Input: part model. Units: mm. Frame: model coordinates. Coordinates: 2 decimals unless noted, no trailing zeros. Loops run counter-clockwise (first coordinate to the right, second up) from the corner with the lowest first, then second, coordinate; pieces in that order, holes last. Notation, with made-up numbers: (71.5, 4) -> (97.5, 4) arc R22 cw to (97.5, 43) -> close; hole circle Ø3 at (-28.5, 8). An arc over 180 degrees is marked (long way). Put each result on its own line as item: value. Start each with the question number.
1) Cut plane B-B (z = 32). Return the cut outline in (x, y), plus the area to 3 significant figures.
2) Cut plane A-A (x = -163). Return the cut outline in (y, z).
3) Contact query for flat-ended pins moving along their axis: P1, Ø7.5, axis at x = -13.74, y = 0, coming from the -Z side; P2, Ø7.5, axis at x = 247.5, y = 2.5, coming from the -Z side; P3, Ø3, axis at x = 134.5, z = 18, coming from the -Y side. Output: stop coordinate, or through.
4) Material intervals for L1, parallel to X at y = 32.5, z = 9.5; L2, parallel to Y at x = 300, z = 13; L3, parallel to X at y = 44, z = 22.5, sorted ascending.
from build123d import *

# Parameters (mm, degrees)
SKETCH1_W           = 965.2
SKETCH1_H           = 127
BOSS_EXTRUDE1_DEPTH = 44.45
FILLET1_R           = 31.75
FILLET2_R           = 31.75
FILLET3_R           = 31.75
SKETCH6_R           = 4.7625
CUT_EXTRUDE1_DEPTH  = 25.4


with BuildPart() as part:
    # Sketch1 → Boss-Extrude1 (new, symmetric)
    with BuildSketch(Plane.XY):
        Rectangle(SKETCH1_W, SKETCH1_H)
    extrude(amount=BOSS_EXTRUDE1_DEPTH, both=True)

    # Fillet1
    fillet1_edges = [part.edges().sort_by_distance(p)[0] for p in [
        (0, -63.5, 44.45),
        (0, 63.5, 44.45),
    ]]
    fillet(fillet1_edges, radius=FILLET1_R)

    # Fillet2
    fillet2_edges = [part.edges().sort_by_distance(p)[0] for p in [
        (-482.6, 0, 44.45),
        (-482.6, -63.5, -15.875),
        (-482.6, 63.5, -15.875),
        (-482.6, 54.200640303, 35.150640303),
        (-482.6, -54.200640303, 35.150640303),
    ]]
    fillet(fillet2_edges, radius=FILLET2_R)

    # Fillet3
    fillet3_edges = [part.edges().sort_by_distance(p)[0] for p in [
        (482.6, 0, 44.45),
        (482.6, 63.5, -15.875),
        (482.6, -63.5, -15.875),
        (482.6, 54.200640303, 35.150640303),
        (482.6, -54.200640303, 35.150640303),
    ]]
    fillet(fillet3_edges, radius=FILLET3_R)

    # Sketch6 → Cut-Extrude1 (cut)
    with BuildSketch(Plane(origin=(0, 0, -44.45), x_dir=(-1, 0, 0), z_dir=(0, 0, -1))):
        with Locations((-11.655611638, 0)):
            Circle(SKETCH6_R)
        with Locations((13.744388362, 0)):
            Circle(SKETCH6_R)
        with Locations((-271.716271796, 0.118953538)):
            Circle(SKETCH6_R)
        with Locations((-246.316271796, 0.118953538)):
            Circle(SKETCH6_R)
        with Locations(Location((246.316271796, 0.118953538, 0), (0, 0, 180))):
            Circle(SKETCH6_R)
        with Locations(Location((271.716271796, 0.118953538, 0), (0, 0, 180))):
            Circle(SKETCH6_R)
    extrude(amount=-CUT_EXTRUDE1_DEPTH, mode=Mode.SUBTRACT)


solid = part.part
Results found:
1. outline: (-476.06, -31.75) arc R25.21 ccw to (-450.85, -56.96) -> (450.85, -56.96) arc R25.21 ccw to (476.06, -31.75) -> (476.06, 31.75) arc R25.21 ccw to (450.85, 56.96) -> (-450.85, 56.96) arc R25.21 ccw to (-476.06, 31.75) -> close
1. area: 108,000 mm2
2. outline: (-63.5, -44.45) -> (63.5, -44.45) -> (63.5, 12.7) arc R31.75 ccw to (31.75, 44.45) -> (-31.75, 44.45) arc R31.75 ccw to (-63.5, 12.7) -> close
3. P1: stops at z = -19.05
3. P2: stops at z = -44.45
3. P3: stops at y = -63.27
4. L1: x = -482.59 to 482.59
4. L2: y = -63.5 to 63.5
4. L3: x = -478.45 to 478.45
